Read the model definition and answer for the solid it produces. Units are mm, in the model's axes. A direction names the side the tool comes from. Give positions to 0.01 mm unless a question says otherwise; leave off trailing zeros. Loops run counter-clockwise (first coordinate to the right, second up) from the corner with the lowest first, then second, coordinate; pieces in that order, holes last. Notation, with made-up numbers: (-2, -18.5) - (50, -18.5) arc R26 cw to (50, 16.5) - close; hole circle Ø2 at (71.5, 34.5). An arc over 180 degrees is marked (long way). Write item = value, one per line.
```python
from build123d import *

# Parameters (mm, degrees)
BOSS_EXTRUDE1_DEPTH      = 30
BOSS_EXTRUDE1_DEPTH_BACK = 30
SKETCH1_W                = 950
SKETCH1_H                = 750
SKETCH1_W_2              = 850
SKETCH1_H_2              = 650
SKETCH3_R                = 25
BOSS_EXTRUDE2_DEPTH      = 118.75
SKETCH4_R                = 27.5
CUT_EXTRUDE2_DEPTH       = 85


with BuildPart() as part:
    # Sketch1 → Boss-Extrude1 (new, two sides: drawn at the far end of the back side and taken through both)
    with BuildSketch(Plane.XY.offset(-BOSS_EXTRUDE1_DEPTH_BACK)):
        Rectangle(SKETCH1_W, SKETCH1_H)
        Rectangle(SKETCH1_W_2, SKETCH1_H_2, mode=Mode.SUBTRACT)
    extrude(amount=BOSS_EXTRUDE1_DEPTH + BOSS_EXTRUDE1_DEPTH_BACK)

    # Sketch3 → Boss-Extrude2 (add)
    with BuildSketch(Plane(origin=(475, 0, 0), x_dir=(0, 0, -1), z_dir=(1, 0, 0))):
        with Locations(Location((0, 0, 0), (0, 0, 270))):
            Circle(SKETCH3_R)
    boss_extrude2 = extrude(amount=BOSS_EXTRUDE2_DEPTH)

    # Mirror2: Boss-Extrude2 across plane
    add(boss_extrude2.mirror(Plane(origin=(0, 0, 0), x_dir=(0, 0, 1), z_dir=(1, 0, 0))))

    # Sketch4 → Cut-Extrude2 (cut)
    with BuildSketch(Plane.XZ.offset(-325)):
        with Locations(Location((0, 0, 0), (0, 0, 270))):
            Circle(SKETCH4_R)
    cut_extrude2 = extrude(amount=-CUT_EXTRUDE2_DEPTH, mode=Mode.SUBTRACT)

    # Mirror3: Cut-Extrude2 across plane
    add(cut_extrude2.mirror(Plane.ZX), mode=Mode.SUBTRACT)


solid = part.part
```
1) Each of these flat-tipped pins is pushed along its axis until it touches: P1, Ø4, axis at y = 212.5, z = 16.5, coming from the -X side; P2, Ø18, axis at y = 85, z = 8, coming from the +X side. Where does it stop, or does it pass through?
Output:
P1 = -475
P2 = 475
2) A cutting plane is placed at B-B on y = 0. Determine the outline of the cut face in (x, z), then the cut area to 3 significant figures.
Output:
outline = (-593.75, -25) - (-475, -25) - (-475, -30) - (-425, -30) - (-425, 30) - (-475, 30) - (-475, 25) - (-593.75, 25) - close; (425, -30) - (475, -30) - (475, -25) - (593.75, -25) - (593.75, 25) - (475, 25) - (475, 30) - (425, 30) - close
area = 17,900 mm²
3) The mould has two halves that part along Y. Classify faces 4 (the face through (-24.397, 349.65, -12.69)), 5 (the face through (-425, -5, 0)), 6 (the face through (533.544, -23.846, -7.509)): pulls with the +Y half, pulls with the -Y half, needs draft (parallel to the pull), parting line crosses it, or undercut.
Output:
face_4 = needs draft
face_5 = undercut
face_6 = parting line crosses it
4) Find the intervals of material crossed by probe 1 along X at (y, z) = (211, -23.5); probe 2 along X at (y, z) = (-339, 0); probe 3 along Y at (x, z) = (-332.5, 17), in increasing order.
Output:
probe_1 = -475 to -425, 425 to 475
probe_2 = -475 to -27.5, 27.5 to 475
probe_3 = -375 to -325, 325 to 375
5) A cutting plane is placed at A-A on x = -215.5. Determine the outline of the cut face in (y, z), then the cut area to 3 significant figures.
Output:
outline = (-375, -30) - (-325, -30) - (-325, 30) - (-375, 30) - close; (325, -30) - (375, -30) - (375, 30) - (325, 30) - close
area = 6,000 mm²
6) A cutting plane is placed at D-D on x = 0. Determine the outline of the cut face in (y, z), then the cut area to 3 significant figures.
Output:
outline = (-375, -30) - (-325, -30) - (-325, -27.5) - (-375, -27.5) - close; (-375, 27.5) - (-325, 27.5) - (-325, 30) - (-375, 30) - close; (325, -30) - (375, -30) - (375, -27.5) - (325, -27.5) - close; (325, 27.5) - (375, 27.5) - (375, 30) - (325, 30) - close
area = 500 mm²
7) A tool of negligible diameter and unlimited length cuts with its end or side. For faces 1 (the face through (-7, -375, -27)), 2 (the face through (-533.544, -23.846, -7.509)), 3 (the face through (-6, -325, -27)), from which of +Z, -Z, +X, -X, +Y, -Y can it reach the whole face along a straight path? Write none if from no direction.
Output:
face_1 = +Z, -Z, +X, -X, -Y
face_2 = -X
face_3 = +Z, -Z
8) A cutting plane is placed at C-C on z = 0. Determine the outline of the cut face in (x, y), then the cut area to 3 significant figures.
Output:
outline = (-593.75, -25) - (-475, -25) - (-475, -375) - (-27.5, -375) - (-27.5, -325) - (-425, -325) - (-425, 325) - (-27.5, 325) - (-27.5, 375) - (-475, 375) - (-475, 25) - (-593.75, 25) - close; (27.5, -375) - (475, -375) - (475, -25) - (593.75, -25) - (593.75, 25) - (475, 25) - (475, 375) - (27.5, 375) - (27.5, 325) - (425, 325) - (425, -325) - (27.5, -325) - close
area = 166,000 mm²
